CAD build for the part. Positions are in the model's coordinates, mm. A direction names the side the tool comes from. Coordinates: 2 decimals unless noted, no trailing zeros. Order: outer loops, then holes, each group sorted by start corner. A loop starts at its lowest first (then second) coordinate and runs counter-clockwise, first axis right, second up. Notation, with made-up numbers: M 20.5,15 L 33.5,15 A21 cw 33.5,23 Z; hole C 24.5,59.5 d7. An arc over 180 degrees is marked long. Write item = value, one per line.
from build123d import *

# Parameters (mm, degrees)
F0_W     = 80
F0_H     = 63
F1_DEPTH = 15.5
F3_DEPTH = 77.25
F4_R     = 5.08
F5_R     = 1
F6_DEPTH = 98.552


with BuildPart() as f1:
    # F0 (on Top) → F1 (new body)
    with BuildSketch(Plane.XY):
        with Locations((8.368649, -7.845957)):
            Rectangle(F0_W, F0_H)
    extrude(amount=F1_DEPTH)

    # F2 (on face) → F3 (cut)
    with BuildSketch(Plane.YZ.offset(48.368649)):
        with BuildLine():
            Line((-31.595957, 2.5), (-7.845957, 2.5))
            Line((-7.845957, 2.5), (15.904043, 2.5))
            ThreePointArc((15.904043, 2.5), (19.616353, 4.037689), (21.154043, 7.75))
            ThreePointArc((21.154043, 7.75), (19.616353, 11.462311), (15.904043, 13))
            Line((15.904043, 13), (-7.845957, 13))
            Line((-7.845957, 13), (-31.595957, 13))
            ThreePointArc((-31.595957, 13), (-35.308268, 11.462311), (-36.845957, 7.75))
            ThreePointArc((-36.845957, 7.75), (-35.308268, 4.037689), (-31.595957, 2.5))
        make_face()
    extrude(amount=-F3_DEPTH, mode=Mode.SUBTRACT)

    # F4
    f4_edges = [f1.edges().sort_by_distance(p)[0] for p in [
        (8.368649, -39.345957, 15.5),
        (8.368649, -39.345957, 0),
        (8.368649, 23.654043, 15.5),
        (8.368649, 23.654043, 0),
    ]]
    fillet(f4_edges, radius=F4_R)

    # F5
    f5_edges = [f1.edges().sort_by_distance(p)[0] for p in [
        (-31.631351, -7.845957, 15.5),
        (48.368649, -7.845957, 15.5),
    ]]
    fillet(f5_edges, radius=F5_R)

    # F2 (on face) → F6 (cut)
    with BuildSketch(Plane.YZ.offset(48.368649)):
        with BuildLine():
            ThreePointArc((15.904043, 13), (19.616353, 11.462311), (21.154043, 7.75))
            Line((21.154043, 7.75), (23.654043, 7.75))
            Line((23.654043, 7.75), (23.654043, 15.5))
            Line((23.654043, 15.5), (-39.345957, 15.5))
            Line((-39.345957, 15.5), (-39.345957, 7.75))
            Line((-39.345957, 7.75), (-36.845957, 7.75))
            ThreePointArc((-36.845957, 7.75), (-35.308268, 11.462311), (-31.595957, 13))
            Line((-31.595957, 13), (-7.845957, 13))
            Line((-7.845957, 13), (15.904043, 13))
        make_face()
    extrude(amount=-F6_DEPTH, mode=Mode.SUBTRACT)


solid = f1.part
(1) Slice it at A-A, the plane x = 2. Write the cut outline in (y, z), then the cut area to 3 significant figures.
Evaluation:
outline = M -39.35,5.08 A5.08 ccw -34.27,0 L 18.57,0 A5.08 ccw 23.65,5.08 L 23.65,7.75 L 21.15,7.75 A5.25 cw 15.9,2.5 L -31.6,2.5 A5.25 cw -36.85,7.75 L -39.35,7.75 Z
area = 185 mm²
(2) Tool access for faces 4 (the face through (8.91, -37.9, 1.53)), 5 (the face through (10.28, -35.35, 4.08)): list every direction of +Z, -Z, +X, -X, +Y, -Y with a clear straight run to the whole face (end or side of a thin tool).
Evaluation:
face_4 = -Z, +X, -X, -Y
face_5 = +Z, +X
(3) Pull direction Y, two halves, no side cores. Call faces 1 (the face through (10.28, 19.58, 4)), 2 (the face through (-30, -8, 13)), 3 (the face through (8, -39.346, 6)): +Y half, -Y half, draft (parallel to the pull), parting line (faces both ways), or undercut.
Evaluation:
face_1 = undercut
face_2 = draft
face_3 = -Y half
(4) Slice it at C-C, the plane z = 10. Write the cut outline in (x, y), then the cut area to 3 significant figures.
Evaluation:
outline = M -31.63,-36.34 L -28.88,-36.34 L -28.88,20.65 L -31.63,20.65 Z
area = 157 mm²
(5) Slice it at B-B, the plane y = -26.5. Write the cut outline in (x, z), then the cut area to 3 significant figures.
Evaluation:
outline = M -31.63,1 A1 ccw -30.63,0 L 47.37,0 A1 ccw 48.37,1 L 48.37,2.5 L -28.88,2.5 L -28.88,13 L -31.63,13 Z
area = 228 mm²
(6) Pin check, flat tips, straight feed: pin 1 Ø24 at (x, y) = (-6, -5) entering from +Z; pin 2 Ø5.5 at (y, z) = (-18.5, 9) entering from +X; pin 3 Ø2 at (x, y) = (11, 22) entering from +Z. Stop position of each tip, or through.
Evaluation:
pin_1 = 2.5
pin_2 = -28.88
pin_3 = 7.75
(7) Wall check: line 1 (Z direction, x = 10.5, y = -25.5); line 2 (X direction, y = -17, z = 11.5); line 3 (Y direction, x = 1, z = 3). Give the ranges that are in metal, low to high. Write a range as from..to.
Evaluation:
line_1 = 0..2.5
line_2 = -31.63..-28.88
line_3 = -38.9..-33.83, 18.14..23.21
